The model under review builds one solid part; all positions refer to its coordinate system, in mm. A direction names the side the tool comes from. Coordinates: 2 decimals unless noted, no trailing zeros. Order: outer loops, then holes, each group sorted by start corner. A loop starts at its lowest first (then second) coordinate and runs counter-clockwise, first axis right, second up. Notation, with made-up numbers: (-30, -35.75) -> (0, -35.75) arc R32 ccw to (0, 1.25) -> close; hole circle Ø6 at (-17.5, 25.5). An arc over 180 degrees is marked (long way). Put each result on its own line as item: value.
from build123d import *

# Parameters (mm, degrees)
SKETCH1_R                             = 6
SKETCH1_R_2                           = 1.5
DISPLAY_SCREW_PATTERN_DEPTH           = 3
DISPLAY_SCREW_PATTERN_2_DEPTH         = 3
DISPLAY_SCREW_PATTERN_3_DEPTH         = 3
DISPLAY_SCREW_PATTERN_4_DEPTH         = 3
DISPLAY_SCREW_PATTERN_5_DEPTH         = 3
SKETCH2_W                             = 311.1
SKETCH2_H                             = 132.6
SKETCH2_R                             = 4
DISPLAY_BACKPLANE_DEPTH               = 3
BACKPLANE_WEIGHT_REDUCTION_DEPTH      = 203.770122306
BACKPLANE_WEIGHT_REDUCTION_DEPTH_BACK = 203.770122306
SKETCH4_W                             = 311.1
SKETCH4_H                             = 132.6
SKETCH4_W_2                           = 309.1
SKETCH4_H_2                           = 130.6
DISPLAY_OUTSIDE_CRADDLE_DEPTH         = 12


with BuildPart() as part:
    # Sketch1 → Display screw pattern (new body)
    with BuildSketch(Plane.XY):
        Circle(SKETCH1_R)
        Circle(SKETCH1_R_2, mode=Mode.SUBTRACT)
    extrude(amount=DISPLAY_SCREW_PATTERN_DEPTH)



with BuildPart() as body_2:
    # Sketch1 → Display screw pattern 2 (new body)
    with BuildSketch(Plane.XY):
        with Locations((-106.24, 18.83)):
            Circle(SKETCH1_R)
        with Locations((-106.24, 18.83)):
            Circle(SKETCH1_R_2, mode=Mode.SUBTRACT)
    extrude(amount=DISPLAY_SCREW_PATTERN_2_DEPTH)


with BuildPart() as body_3:
    # Sketch1 → Display screw pattern 3 (new body)
    with BuildSketch(Plane.XY):
        with Locations((147.61, 18.83)):
            Circle(SKETCH1_R)
        with Locations((147.61, 18.83)):
            Circle(SKETCH1_R_2, mode=Mode.SUBTRACT)
    extrude(amount=DISPLAY_SCREW_PATTERN_3_DEPTH)


with BuildPart() as body_4:
    # Sketch1 → Display screw pattern 4 (new body)
    with BuildSketch(Plane.XY):
        with Locations((-121.24, -91.25)):
            Circle(SKETCH1_R)
        with Locations((-121.24, -91.25)):
            Circle(SKETCH1_R_2, mode=Mode.SUBTRACT)
    extrude(amount=DISPLAY_SCREW_PATTERN_4_DEPTH)


with BuildPart() as body_5:
    # Sketch1 → Display screw pattern 5 (new body)
    with BuildSketch(Plane.XY):
        with Locations((162.61, -91.25)):
            Circle(SKETCH1_R)
        with Locations((162.61, -91.25)):
            Circle(SKETCH1_R_2, mode=Mode.SUBTRACT)
    extrude(amount=DISPLAY_SCREW_PATTERN_5_DEPTH)


with BuildPart() as part_1:
    add(part.part)

    add(body_2.part)  # Display backplane merges body 2

    add(body_3.part)  # Display backplane merges body 3

    add(body_4.part)  # Display backplane merges body 4

    add(body_5.part)  # Display backplane merges body 5
    # Sketch2 → Display backplane (add)
    with BuildSketch(Plane(origin=(0, 0, 0), x_dir=(-1, 0, 0), z_dir=(0, 0, -1))):
        with Locations((-20.21, -34.77)):
            Rectangle(SKETCH2_W, SKETCH2_H)
        with Locations((106.24, 18.83)):
            Circle(SKETCH2_R, mode=Mode.SUBTRACT)
        Circle(SKETCH2_R, mode=Mode.SUBTRACT)
        with Locations((121.24, -91.25)):
            Circle(SKETCH2_R, mode=Mode.SUBTRACT)
        with Locations((-147.61, 18.83)):
            Circle(SKETCH2_R, mode=Mode.SUBTRACT)
        with Locations((-162.61, -91.25)):
            Circle(SKETCH2_R, mode=Mode.SUBTRACT)
    extrude(amount=DISPLAY_BACKPLANE_DEPTH)

    # Sketch3 → Backplane weight reduction (cut, two sides: drawn at the far end of the back side and taken through both)
    with BuildSketch(Plane.XY.offset(-BACKPLANE_WEIGHT_REDUCTION_DEPTH_BACK)):
        with BuildLine():
            Line((162.61, -7.17), (162.61, -67.25))
            ThreePointArc((162.61, -67.25), (160.930502943, -72.797001962), (156.456153846, -76.480769231))
            ThreePointArc((156.456153846, -76.480769231), (151.296291501, -79.936291501), (147.840769231, -85.096153846))
            ThreePointArc((147.840769231, -85.096153846), (144.157001962, -89.570502943), (138.61, -91.25))
            Line((138.61, -91.25), (-97.24, -91.25))
            ThreePointArc((-97.24, -91.25), (-102.787001962, -89.570502943), (-106.470769231, -85.096153846))
            ThreePointArc((-106.470769231, -85.096153846), (-109.926291501, -79.936291501), (-115.086153846, -76.480769231))
            ThreePointArc((-115.086153846, -76.480769231), (-119.560502943, -72.797001962), (-121.24, -67.25))
            Line((-121.24, -67.25), (-121.24, -7.17))
            ThreePointArc((-121.24, -7.17), (-118.311067812, -0.098932188), (-111.24, 2.83))
            Line((-111.24, 2.83), (-106.24, 2.83))
            ThreePointArc((-106.24, 2.83), (-97.36479686, 5.517195291), (-91.470769231, 12.676153846))
            ThreePointArc((-91.470769231, 12.676153846), (-87.787001962, 17.150502943), (-82.24, 18.83))
            Line((-82.24, 18.83), (-21, 18.83))
            ThreePointArc((-21, 18.83), (-13.928932188, 15.901067812), (-11, 8.83))
            Line((-11, 8.83), (-11, 0))
            ThreePointArc((-11, 0), (0, -11), (11, 0))
            Line((11, 0), (11, 8.83))
            ThreePointArc((11, 8.83), (13.928932188, 15.901067812), (21, 18.83))
            Line((21, 18.83), (123.61, 18.83))
            ThreePointArc((123.61, 18.83), (129.157001962, 17.150502943), (132.840769231, 12.676153846))
            ThreePointArc((132.840769231, 12.676153846), (138.73479686, 5.517195291), (147.61, 2.83))
            Line((147.61, 2.83), (152.61, 2.83))
            ThreePointArc((152.61, 2.83), (159.681067812, -0.098932188), (162.61, -7.17))
        make_face()
    extrude(amount=BACKPLANE_WEIGHT_REDUCTION_DEPTH + BACKPLANE_WEIGHT_REDUCTION_DEPTH_BACK, mode=Mode.SUBTRACT)

    # Sketch4 → Display outside craddle (add)
    with BuildSketch(Plane(origin=(0, 0, -3), x_dir=(-1, 0, 0), z_dir=(0, 0, -1))):
        with Locations((-20.21, -34.77)):
            Rectangle(SKETCH4_W, SKETCH4_H)
        with Locations((-20.21, -34.77)):
            Rectangle(SKETCH4_W_2, SKETCH4_H_2, mode=Mode.SUBTRACT)
    extrude(amount=DISPLAY_OUTSIDE_CRADDLE_DEPTH)


solid = part_1.part
Item 1: Consider section C-C on z = -10. Write out the cut boundary in (x, y), and give its area (3 significant figures).
Answers below:
outline: (-135.34, -101.07) -> (175.76, -101.07) -> (175.76, 31.53) -> (-135.34, 31.53) -> close; hole (-134.34, -100.07) -> (174.76, -100.07) -> (174.76, 30.53) -> (-134.34, 30.53) -> close
area: 883 mm^2
Item 2: For pin 1 Ø9 at (x, y) = (-121.24, -91.25) entering from -Z; pin 2 Ø2.5 at (x, y) = (0.5, 2) entering from -Z, all flat-tipped, find the tip position at first contact; note any pin that passes through.
Answers below:
pin 1: z = -3
pin 2: z = 0
Item 3: For faces 1 (the cylindrical face through (-118.39, -0.18, -1.52)), 2 (the cylindrical face through (-120.373, -95.155, -1.479)), 3 (the flat face through (175.76, -36, -7)), list the 3-axis set-ups (+Z, -Z, +X, -X, +Y, -Y) from which the entire face can be reached by the end or side of a thin tool; tool diameter is ignored.
Answers below:
face 1: +Z, -Z
face 2: -Z
face 3: +Z, -Z, +X, +Y, -Y
Item 4: Consider section B-B on x = 40. Write out the cut boundary in (y, z).
Answers below:
outline: (-101.07, -15) -> (-100.07, -15) -> (-100.07, -3) -> (-91.25, -3) -> (-91.25, 0) -> (-101.07, 0) -> close; (18.83, -3) -> (30.53, -3) -> (30.53, -15) -> (31.53, -15) -> (31.53, 0) -> (18.83, 0) -> close
Item 5: For line 1 (Y direction, x = 0, z = -1.65); line 2 (Y direction, x = 132.5, z = -14); line 3 (X direction, y = -85.5, z = -3.75), list the stretches that pass through material, from the lowest coordinate up. Write a range as from..to.
Answers below:
line 1: -101.07..-91.25, -11..-4, 4..31.53
line 2: -101.07..-100.07, 30.53..31.53
line 3: -135.34..-134.34, 174.76..175.76
Item 6: Consider section A-A on y = -17.5. Write out the cut boundary in (x, z), and give its area (3 significant figures).
Answers below:
outline: (-135.34, -15) -> (-134.34, -15) -> (-134.34, -3) -> (-121.24, -3) -> (-121.24, 0) -> (-135.34, 0) -> close; (162.61, -3) -> (174.76, -3) -> (174.76, -15) -> (175.76, -15) -> (175.76, 0) -> (162.61, 0) -> close
area: 106 mm^2
Item 7: Mouldability with a two-part tool opening along X and no side actions: class faces 4 (the flat face through (22, -101.07, -7)), 5 (the cylindrical face through (-6, 0, 1)), 6 (the flat face through (22, 30.53, -9)) as +X half, -X half, draft (parallel to the pull), parting line (faces both ways), or undercut.
Answers below:
face 4: draft
face 5: parting line
face 6: undercut
